The listing builds one solid part. Answer for the finished solid, in the listing's coordinates (mm). Round coordinates to 2 decimals unless told otherwise and drop trailing zeros. Write each loop counter-clockwise with the first axis right and the second up, starting at its lowest first coordinate (ties: lowest second). Pieces come first, ordered by that corner, then holes.
from build123d import *

# Parameters (mm, degrees)
F1_DEPTH = 147.9502767324


with BuildPart() as f1:
    # F0 (on Top) → F1 (new body)
    with BuildSketch(Plane.XY):
        with BuildLine():
            ThreePointArc((-87.9484422868, -78.1952069234), (-228.9705848103, -86.1188770419), (-144.926183088, -199.6378964581))
            ThreePointArc((-144.926183088, -199.6378964581), (-141.9776426647, -182.625293005), (-135.4781136343, -166.6290844149))
            ThreePointArc((-135.4781136343, -166.6290844149), (-143.1221520937, -105.5311323371), (-87.9484422868, -78.1952069234))
        make_face()
        with BuildLine():
            ThreePointArc((-43.1303394705, -130.6995274151), (-43.1637393197, -128.8153342329), (-43.2638969004, -126.9335085352))
            ThreePointArc((-43.2638969004, -126.9335085352), (-59.6405921047, -124.2616153411), (-76.2175991553, -124.9950976526))
            ThreePointArc((-76.2175991553, -124.9950976526), (-85.0850207305, -157.1491742454), (-106.2593539774, -182.9205424373))
            ThreePointArc((-106.2593539774, -182.9205424373), (-62.407597495, -171.6638621544), (-43.1303394705, -130.6995274151))
        make_face()
        with BuildLine():
            ThreePointArc((-135.4781136343, -166.6290844149), (-141.9776426647, -182.625293005), (-144.926183088, -199.6378964581))
            ThreePointArc((-144.926183088, -199.6378964581), (-124.4762204529, -193.8617677231), (-106.2593539774, -182.9205424373))
            ThreePointArc((-106.2593539774, -182.9205424373), (-122.1835688251, -177.1329724297), (-135.4781136343, -166.6290844149))
        make_face()
        with BuildLine():
            ThreePointArc((-76.2175991553, -124.9950976526), (-59.6405921047, -124.2616153411), (-43.2638969004, -126.9335085352))
            ThreePointArc((-43.2638969004, -126.9335085352), (-57.1072322193, -94.7723104014), (-87.9484422868, -78.1952069234))
            ThreePointArc((-87.9484422868, -78.1952069234), (-79.099972808, -98.3765624175), (-76.0744358047, -120.20380795))
            ThreePointArc((-76.0744358047, -120.20380795), (-76.1102346274, -122.6005219901), (-76.2175991553, -124.9950976526))
        make_face()
        with BuildLine():
            ThreePointArc((-135.4781136343, -166.6290844149), (-110.7796966213, -138.7922639194), (-76.2175991553, -124.9950976526))
            ThreePointArc((-76.2175991553, -124.9950976526), (-76.1102346274, -122.6005219901), (-76.0744358047, -120.20380795))
            ThreePointArc((-76.0744358047, -120.20380795), (-79.099972808, -98.3765624175), (-87.9484422868, -78.1952069234))
            ThreePointArc((-87.9484422868, -78.1952069234), (-143.1221520937, -105.5311323371), (-135.4781136343, -166.6290844149))
        make_face()
        with BuildLine():
            ThreePointArc((-144.926183088, -199.6378964581), (-66.9805164151, -285.5076041639), (16.3334276456, -204.835921526))
            ThreePointArc((16.3334276456, -204.835921526), (-0.2745731056, -155.7935239428), (-43.2638969004, -126.9335085352))
            ThreePointArc((-43.2638969004, -126.9335085352), (-43.1637393197, -128.8153342329), (-43.1303394705, -130.6995274151))
            ThreePointArc((-43.1303394705, -130.6995274151), (-62.407597495, -171.6638621544), (-106.2593539774, -182.9205424373))
            ThreePointArc((-106.2593539774, -182.9205424373), (-124.4762204529, -193.8617677231), (-144.926183088, -199.6378964581))
        make_face()
    extrude(amount=F1_DEPTH)


solid = f1.part
1. For a pull along X with two mould halves and no side action, classify faces 1 (the face through (-121.975, -177.249, 72.939)), 2 (the face through (-112, -134, 147.95)), 3 (the face through (-56.771, -95.142, 72.939)) as released by +X, released by -X, zero draft, split by the parting line, or undercut.
Geometry says:
face 1: undercut
face 2: zero draft
face 3: released by +X
2. Section A-A on x = -129.5 is taken. Determine the outline of the cut face in (y, z).
Geometry says:
outline: (-252.52, 0) - (-172.22, 0) - (-172.22, 147.95) - (-252.52, 147.95) - close; (-157.15, 0) - (-44.57, 0) - (-44.57, 147.95) - (-157.15, 147.95) - close
3. Section D-D on x = -156 is taken. Determine the outline of the cut face in (y, z).
Geometry says:
outline: (-200.45, 0) - (-39.96, 0) - (-39.96, 147.95) - (-200.45, 147.95) - close
4. Section B-B on z = 137 is taken. Determine the outline of the cut face in (x, y).
Geometry says:
outline: (-144.93, -199.64) arc R80.71 ccw (long way) to (-43.26, -126.93) arc R53.16 ccw to (-87.95, -78.2) arc R80.25 ccw (long way) to start; hole (-135.48, -166.63) arc R53.16 ccw to (-106.26, -182.92) arc R80.25 ccw to (-76.22, -125) arc R80.71 ccw to start
5. Given pin 1 (4 mm diameter, centred on x = -70.5, z = 62.5, fed in from +Y); pin 2 (1.5 mm diameter, centred on x = -112, z = 113, fed in from +Y); pin 3 (2 mm diameter, centred on x = -97, z = 116, fed in from -Y), each flat-ended and moving along its own axis, determine where each tip first touches the part or whether it passes through.
Geometry says:
pin 1: stops at y = -83.16
pin 2: stops at y = -52.82
pin 3: stops at y = -279.1
6. Section C-C on y = -70 is taken. Determine the outline of the cut face in (x, z).
Geometry says:
outline: (-218.93, 0) - (-93.72, 0) - (-93.72, 147.95) - (-218.93, 147.95) - close
7. Straight lines are drawn through the part: line 1 along Y through (x, z) = (-156, 106); line 2 along X through (y, z) = (-155, 43); line 3 along Y through (x, z) = (-181, 131). For each, find the intervals that lie inside material, in ascending order.
Geometry says:
line 1: y = -200.45 to -39.96
line 2: x = -228.63 to -127.87, -84.01 to -0.89
line 3: y = -196.56 to -43.85
